For this review, use the dimensioned drawing (mm, ordinates from the lowest corner) and the shaded views. A direction names the side the tool comes from. Give positions to 0.01 mm unless a question says otherwise; leave off trailing zeros. Write each loop counter-clockwise with the first axis right and the second up, starting at its lowest first coordinate (ties: lowest second). Pieces come first, ordered by that corner, then holes.
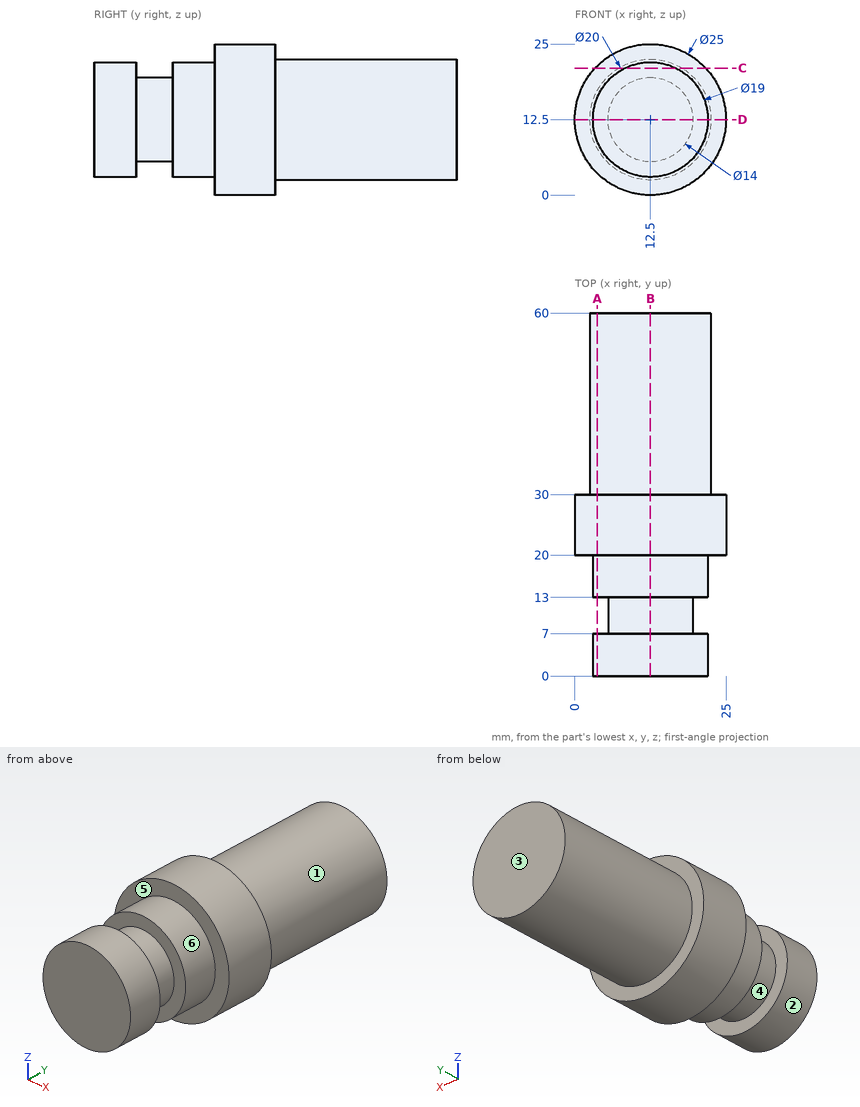
(1) Clearance check with flat-ended pins moving along their axes: pin 1 Ø3 at (x, z) = (10, 11.5) entering from -Y; pin 2 Ø6 at (x, y) = (17, 10.5) entering from +Z; pin 3 Ø6 at (y, z) = (15.5, 22) entering from -X; pin 4 Ø12 at (y, z) = (31.5, 22) entering from +X. State where each tip first meets the part, or that it passes through.
(2) We need section C-C (z = 21). Write out the cut boundary in (x, y), and give its area (3 significant figures).
(3) We need section A-A (x = 3.75). Write out the cut boundary in (y, z).
(4) The part is to be moulded in two halves that separate along Y. For the marked faces 4, 5 and 6, say which applies: +Y half, -Y half, draft (parallel to the pull), parting line (faces both ways), or undercut.
(5) We need section D-D (z = 12.5). Write out the cut boundary in (x, y), and give its area (3 significant figures).
(6) Tool access review of the marked faces 1, 2 and 3: name each direction out of +Z, -Z, +X, -X, +Y, -Y from which nothing blocks a thin tool from reaching the whole face with its end or side.
(7) We need section B-B (x = 12.5). Write out the cut boundary in (y, z).
(8) For L1, parallel to Y at x = 9.5, z = 20.5; L2, parallel to Y at x = 19.5, z = 21.75; L3, parallel to Z at x = 12, y = 16.5, list the stretches that pass through material, from the lowest coordinate up.
The answers:
1. pin 1: stops at y = 0
1. pin 2: stops at z = 21.57
1. pin 3: stops at x = 5.57
1. pin 4: stops at x = 24.44
2. outline: (3.33, 20) - (8.26, 20) - (8.26, 13) - (16.74, 13) - (16.74, 20) - (21.67, 20) - (21.67, 30) - (17.77, 30) - (17.77, 60) - (7.23, 60) - (7.23, 30) - (3.33, 30) - close; (8.26, 0) - (16.74, 0) - (16.74, 7) - (8.26, 7) - close
2. area: 618 mm2
3. outline: (0, 8.8) - (7, 8.8) - (7, 16.2) - (0, 16.2) - close; (13, 8.8) - (20, 8.8) - (20, 3.57) - (30, 3.57) - (30, 7.66) - (60, 7.66) - (60, 17.34) - (30, 17.34) - (30, 21.43) - (20, 21.43) - (20, 16.2) - (13, 16.2) - close
4. face 4: undercut
4. face 5: -Y half
4. face 6: draft
5. outline: (0, 20) - (3, 20) - (3, 13) - (5.5, 13) - (5.5, 7) - (3, 7) - (3, 0) - (22, 0) - (22, 7) - (19.5, 7) - (19.5, 13) - (22, 13) - (22, 20) - (25, 20) - (25, 30) - (22.5, 30) - (22.5, 60) - (2.5, 60) - (2.5, 30) - (0, 30) - close
5. area: 1,200 mm2
6. face 1: +Y
6. face 2: -Y
6. face 3: +Z, -Z, +X, -X, +Y
7. outline: (0, 3) - (7, 3) - (7, 5.5) - (13, 5.5) - (13, 3) - (20, 3) - (20, 0) - (30, 0) - (30, 2.5) - (60, 2.5) - (60, 22.5) - (30, 22.5) - (30, 25) - (20, 25) - (20, 22) - (13, 22) - (13, 19.5) - (7, 19.5) - (7, 22) - (0, 22) - close
8. L1: y = 0 to 7, 13 to 60
8. L2: y = 20 to 30
8. L3: z = 3.01 to 21.99
